from build123d import *

# Parameters (mm, degrees)
SKETCH1_R           = 33
BOSS_EXTRUDE1_DEPTH = 5
SKETCH2_R           = 2
CUT_EXTRUDE1_DEPTH  = 2.5
FILLET1_R           = 5
SKETCH3_W           = 4
SKETCH3_H           = 5
SKETCH3_W_2         = 5
SKETCH3_H_2         = 4
BOSS_EXTRUDE2_DEPTH = 5
FILLET2_R           = 2.5
SKETCH4_R           = 1
CUT_EXTRUDE2_DEPTH  = 5
SKETCH5_R           = 1
CUT_EXTRUDE3_DEPTH  = 5
SKETCH6_R           = 10
CUT_EXTRUDE4_DEPTH  = 5
FILLET3_R           = 2.5


with BuildPart() as part:
    # Sketch1 → Boss-Extrude1 (new body)
    with BuildSketch(Plane(origin=(0, 0, 0), x_dir=(1, 0, 0), z_dir=(0, 1, 0))):
        with Locations(Location((0, 0, 0), (0, 0, 270))):
            Circle(SKETCH1_R)
    extrude(amount=BOSS_EXTRUDE1_DEPTH)

    # Sketch2 → Cut-Extrude1 (cut)
    with BuildSketch(Plane(origin=(0, 5, 0), x_dir=(1, 0, 0), z_dir=(0, 1, 0))):
        with Locations(Location((-26.719955328, -5.965376271, 0), (0, 0, 270))):
            Circle(SKETCH2_R)
        with Locations(Location((-5.965376271, 26.719955328, 0), (0, 0, 270))):
            Circle(SKETCH2_R)
        with Locations(Location((26.719955328, 5.965376271, 0), (0, 0, 270))):
            Circle(SKETCH2_R)
        with Locations(Location((5.965376271, -26.719955328, 0), (0, 0, 270))):
            Circle(SKETCH2_R)
    extrude(amount=-CUT_EXTRUDE1_DEPTH, mode=Mode.SUBTRACT)

    # Fillet1
    fillet1_edges = [part.edges().sort_by_distance(p)[0] for p in [
        (0, 0, -33),
    ]]
    fillet(fillet1_edges, radius=FILLET1_R - 0.0001)  # a hair under: the kernel refuses the full size

    # Sketch3 → Boss-Extrude2 (add)
    with BuildSketch(Plane.XZ):
        with Locations((0, 22.5)):
            Rectangle(SKETCH3_W, SKETCH3_H)
        with Locations((-22.5, 0)):
            Rectangle(SKETCH3_W_2, SKETCH3_H_2)
        with Locations((22.5, 0)):
            Rectangle(SKETCH3_W_2, SKETCH3_H_2)
        with Locations((0, -22.5)):
            Rectangle(SKETCH3_W, SKETCH3_H)
    extrude(amount=BOSS_EXTRUDE2_DEPTH)

    # Fillet2
    fillet2_edges = [part.edges().sort_by_distance(p)[0] for p in [
        (0, -5, 20),
        (0, -5, 25),
        (25, -5, 0),
        (20, -5, 0),
        (0, -5, -20),
        (0, -5, -25),
        (-25, -5, 0),
        (-20, -5, 0),
    ]]
    fillet(fillet2_edges, radius=FILLET2_R - 0.0001)  # a hair under: the kernel refuses the full size

    # Sketch4 → Cut-Extrude2 (cut)
    with BuildSketch(Plane(origin=(0, 0, -2), x_dir=(-1, 0, 0), z_dir=(0, 0, -1))):
        with Locations((22.5, -2.5)):
            Circle(SKETCH4_R)
        with Locations((-22.354219449, -2.5)):
            Circle(SKETCH4_R)
    extrude(amount=-CUT_EXTRUDE2_DEPTH, mode=Mode.SUBTRACT)

    # Sketch5 → Cut-Extrude3 (cut)
    with BuildSketch(Plane.ZY.offset(2)):
        with Locations((22.5, -2.5)):
            Circle(SKETCH5_R)
        with Locations((-22.5, -2.5)):
            Circle(SKETCH5_R)
    extrude(amount=-CUT_EXTRUDE3_DEPTH, mode=Mode.SUBTRACT)

    # Sketch6 → Cut-Extrude4 (cut)
    with BuildSketch(Plane.XZ):
        with Locations(Location((0, 0, 0), (0, 0, 270))):
            Circle(SKETCH6_R)
    extrude(amount=-CUT_EXTRUDE4_DEPTH, mode=Mode.SUBTRACT)

    # Fillet3
    fillet3_edges = [part.edges().sort_by_distance(p)[0] for p in [
        (0, 5, 10),
        (0, 0, 10),
    ]]
    fillet(fillet3_edges, radius=FILLET3_R - 0.0001)  # a hair under: the kernel refuses the full size


solid = part.part
Source: CAD feature listing. Evaluate the final solid. Frame: model axes, mm. A direction names the side the tool comes from. Give positions to 0.01 mm unless a question says otherwise; leave off trailing zeros. Order: outer loops, then holes, each group sorted by start corner. A loop starts at its lowest first (then second) coordinate and runs counter-clockwise, first axis right, second up. Notation, with made-up numbers: (88, 30) -> (92, 30) arc R30 cw to (92, 57) -> close; hole circle Ø6 at (-25.75, 20). An arc over 180 degrees is marked (long way). Write item = value, one per line.
Q1. Pull-direction query (Z, two-part tool) for faces 4 (the face through (-27, 2.5, 6)), 5 (the face through (0, -1, 20)), 6 (the face through (-23, -1, -2)), 7 (the face through (0, -1, 25)); classes: released by +Z, released by -Z, zero draft, split by the parting line, or undercut.
Data:
face_4 = undercut
face_5 = undercut
face_6 = released by -Z
face_7 = released by +Z
Q2. Cut plane B-B, the plane y = 4. Output: boundary loops of the cut face in (x, z).
Data:
outline = circle Ø65.8 at (0, 0); hole circle Ø4 at (-26.72, 5.97); hole circle Ø21 at (0, 0); hole circle Ø4 at (-5.97, -26.72); hole circle Ø4 at (5.97, 26.72); hole circle Ø4 at (26.72, -5.97)
Q3. Material intervals for line 1 (Z direction, x = 1.5, y = -2.75); line 2 (Y direction, x = -22.5, z = 0.75); line 3 (Y direction, x = -21.5, z = 13.5), sorted ascending. Write a range as from..to.
Data:
line_1 = -24.99..-23.47, -21.53..-20.01, 20.01..21.53, 23.47..24.99
line_2 = -5..-3.5, -1.5..5
line_3 = 0..5
Q4. Set-up query: faces 1 (the face through (-23, -1, 2)), 2 (the face through (0, -1, -25)), 3 (the face through (20.713, -4.248, 0.028)). Return all of +Z, -Z, +X, -X, +Y, -Y with unobstructed straight access to the full face (end or side cutting, diameter ignored); none if empty.
Data:
face_1 = +Z, +X, -X, -Y
face_2 = -Z, +X, -X, -Y
face_3 = +Z, -Z, -Y
Q5. Cut plane A-A, the plane z = 0. State how many separate pieces and enclosed holes the cut face has, and give its area (3 significant figures).
Data:
separate_pieces = 2
enclosed_holes = 2
area = 252 mm^2
Q6. Pin query (flat end, axial travel): pin 1 (5 mm diameter, centred on x = 16.5, z = 24.5, fed in from -Y); pin 2 (5 mm diameter, centred on x = 7, y = -2, fed in from +Z); pin 3 (2 mm diameter, centred on y = -1.5, z = 1, fed in from -X). Return the tip coordinate at first contact, or that it passes through.
Data:
pin_1 = 0
pin_2 = 29.39
pin_3 = -25
